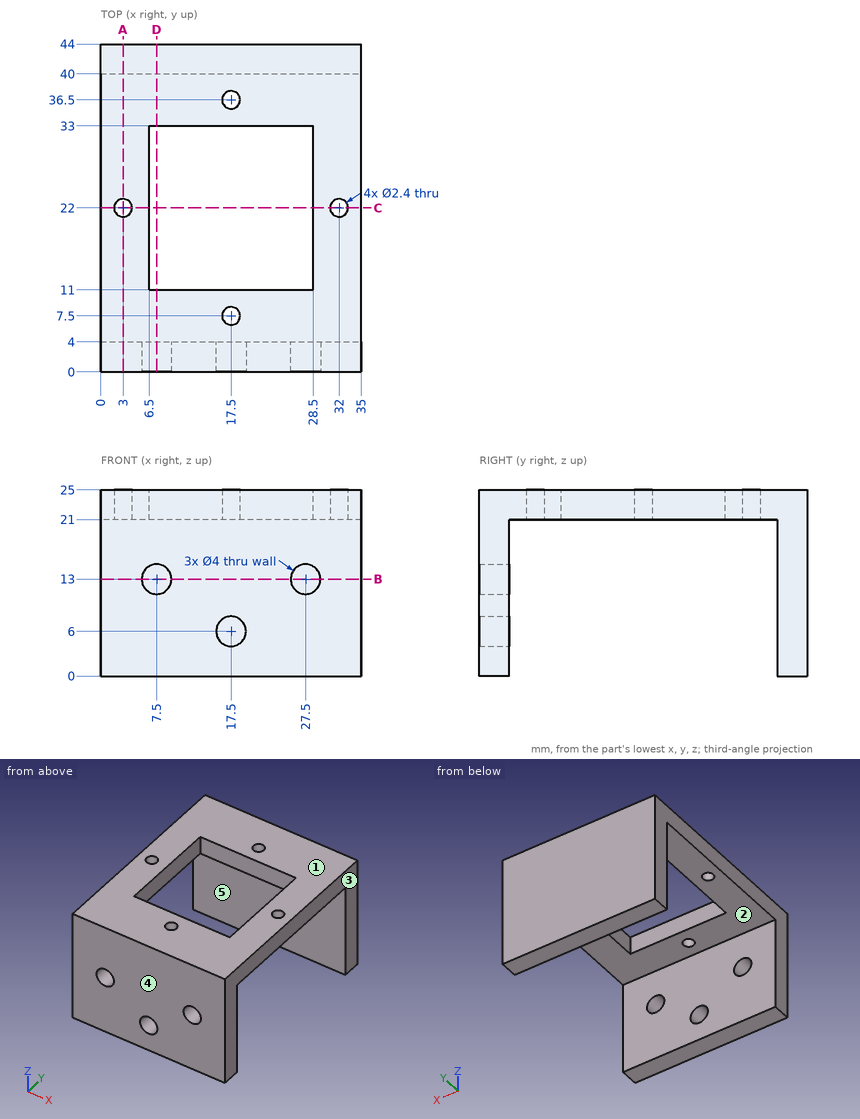
Geometry: see drawing. Coordinates: mm, zero at the bounding-box minimum. A direction names the side the tool comes from. Give positions to 0.01 mm unless a question says otherwise; leave off trailing zeros. Loops run counter-clockwise (first coordinate to the right, second up) from the corner with the lowest first, then second, coordinate; pieces in that order, holes last. Notation, with made-up numbers: (-32.75, 7) -> (25.25, 7) arc R18 ccw to (25.25, 18) -> close; hole circle Ø1 at (0.25, 81). An arc over 180 degrees is marked (long way). Use one line per item in the form item = value.
Item 1: Section query D-D on x = 7.5. Output: boundary loops of the cut face in (y, z).
A:
outline = (0, 0) -> (4, 0) -> (4, 11) -> (0, 11) -> close; (0, 15) -> (4, 15) -> (4, 21) -> (11, 21) -> (11, 25) -> (0, 25) -> close; (33, 21) -> (40, 21) -> (40, 0) -> (44, 0) -> (44, 25) -> (33, 25) -> close
Item 2: Pin query (flat end, axial travel): P1, Ø4, axis at x = 3, y = 22, coming from the -Z side. Return the tip coordinate at first contact, or that it passes through.
A:
P1 = 21
Item 3: Section query A-A on x = 3. Output: boundary loops of the cut face in (y, z), and give its area (3 significant figures).
A:
outline = (0, 0) -> (4, 0) -> (4, 21) -> (20.8, 21) -> (20.8, 25) -> (0, 25) -> close; (23.2, 21) -> (40, 21) -> (40, 0) -> (44, 0) -> (44, 25) -> (23.2, 25) -> close
area = 334 mm^2
Item 4: Section query B-B on z = 13. Output: boundary loops of the cut face in (x, y), and give its area (3 significant figures).
A:
outline = (0, 0) -> (5.5, 0) -> (5.5, 4) -> (0, 4) -> close; (0, 40) -> (35, 40) -> (35, 44) -> (0, 44) -> close; (9.5, 0) -> (25.5, 0) -> (25.5, 4) -> (9.5, 4) -> close; (29.5, 0) -> (35, 0) -> (35, 4) -> (29.5, 4) -> close
area = 248 mm^2
Item 5: Access query for the marked faces 1 and 2. Directions: +Z, -Z, +X, -X, +Y, -Y. A direction counts if a zero-diameter tool reaches every point of the face in a straight line with its end or side. Return the directions, or none.
A:
face_1 = +Z, +X, -X, +Y, -Y
face_2 = -Z, +X, -X
Item 6: Line query: probe 1 along Y at (x, z) = (17.5, 22.65); probe 2 along Y at (x, z) = (2.5, 11); probe 3 along X at (y, z) = (3, 12). Output: solid intervals per line, ascending.
A:
probe_1 = 0 to 6.3, 8.7 to 11, 33 to 35.3, 37.7 to 44
probe_2 = 0 to 4, 40 to 44
probe_3 = 0 to 5.77, 9.23 to 25.77, 29.23 to 35
Item 7: Draft query along Y for the marked faces 3, 4 and 5. Return one class per face: pulls with the +Y half, pulls with the -Y half, needs draft (parallel to the pull), parting line crosses it, or undercut.
A:
face_3 = needs draft
face_4 = pulls with the -Y half
face_5 = undercut
Item 8: Section query C-C on y = 22. Output: boundary loops of the cut face in (x, z), and give its area (3 significant figures).
A:
outline = (0, 21) -> (1.8, 21) -> (1.8, 25) -> (0, 25) -> close; (4.2, 21) -> (6.5, 21) -> (6.5, 25) -> (4.2, 25) -> close; (28.5, 21) -> (30.8, 21) -> (30.8, 25) -> (28.5, 25) -> close; (33.2, 21) -> (35, 21) -> (35, 25) -> (33.2, 25) -> close
area = 32.8 mm^2
